Verification items for the finished model (mm, model axes). Face numbers are marked on the shaded views. Give positions to 0.01 mm unless a question says otherwise; leave off trailing zeros. Write each loop counter-clockwise with the first axis right and the second up, starting at its lowest first coordinate (ties: lowest second). Pieces come first, ordered by that corner, then holes. Notation, with made-up numbers: (-38.5, -26.5) -> (-23.5, -26.5) arc R21 ccw to (-23.5, -10.5) -> close; hole circle Ø5 at (-25.5, 21.25). An arc over 180 degrees is marked (long way). Write item = value, one per line.
from build123d import *

# Parameters (mm, degrees)
BOSS_EXTRUDE1_DEPTH = 6.1
BOSS_EXTRUDE4_START = -5
BOSS_EXTRUDE4_DEPTH = 5
BOSS_EXTRUDE5_START = 5
SKETCH6_R           = 2.75
BOSS_EXTRUDE5_DEPTH = 5
SKETCH7_R           = 2.75
CUT_EXTRUDE1_DEPTH  = 176.534516689


with BuildPart() as part:
    # Sketch4 → Boss-Extrude1 (new body)
    with BuildSketch(Plane.XY):
        with BuildLine():
            Line((2.791805242, 138.827155544), (104.55323324, 91.375022364))
            Line((104.55323324, 91.375022364), (105.415210237, 92.128353131))
            ThreePointArc((105.415210237, 92.128353131), (9.395226761, 139.684393237), (-92.128353131, 105.415210237))
            Line((-92.128353131, 105.415210237), (-91.375022364, 104.55323324))
            Line((-91.375022364, 104.55323324), (2.791805242, 138.827155544))
        make_face()
    extrude(amount=BOSS_EXTRUDE1_DEPTH)

    # Sketch5 → Boss-Extrude4 (add)
    with BuildSketch(Plane.XY.offset(BOSS_EXTRUDE4_START)):
        with BuildLine():
            Line((30.722164617, 125.803015072), (76.622873865, 104.399162835))
            ThreePointArc((76.622873865, 104.399162835), (87.59255508, 95.382358403), (97.50906947, 85.218726646))
            Line((97.50906947, 85.218726646), (105.415210237, 92.128353131))
            ThreePointArc((105.415210237, 92.128353131), (9.395226761, 139.684393237), (-92.128353131, 105.415210237))
            Line((-92.128353131, 105.415210237), (-85.218726646, 97.50906947))
            ThreePointArc((-85.218726646, 97.50906947), (-30.701883618, 125.807966132), (30.722164617, 125.803015072))
        make_face()
    extrude(amount=BOSS_EXTRUDE4_DEPTH)

    # Sketch6 → Boss-Extrude5 (add)
    with BuildSketch(Plane(origin=(0, 0, -5), x_dir=(-1, 0, 0), z_dir=(0, 0, -1)).offset(BOSS_EXTRUDE5_START)):
        with BuildLine():
            Line((-10, 129.5), (10, 129.5))
            Line((10, 129.5), (10, 109.268365161))
            ThreePointArc((10, 109.268365161), (43.208620922, 100.85926186), (72.205596766, 82.619171024))
            Line((72.205596766, 82.619171024), (92.128353131, 105.415210237))
            ThreePointArc((92.128353131, 105.415210237), (-9.395226761, 139.684393237), (-105.415210237, 92.128353131))
            Line((-105.415210237, 92.128353131), (-82.619171024, 72.205596766))
            ThreePointArc((-82.619171024, 72.205596766), (-49.879754516, 97.732214313), (-10, 109.268365161))
            Line((-10, 109.268365161), (-10, 129.5))
        make_face()
        with Locations((54.966796439, 107.162966034)):
            Circle(SKETCH6_R, mode=Mode.SUBTRACT)
    extrude(amount=-BOSS_EXTRUDE5_DEPTH)

    # Sketch7 → Cut-Extrude1 (cut, through all)
    with BuildSketch(Plane.XY):
        with Locations((76.813119358, 91.542310953)):
            Circle(SKETCH7_R)
    extrude(amount=-CUT_EXTRUDE1_DEPTH, mode=Mode.SUBTRACT)


solid = part.part
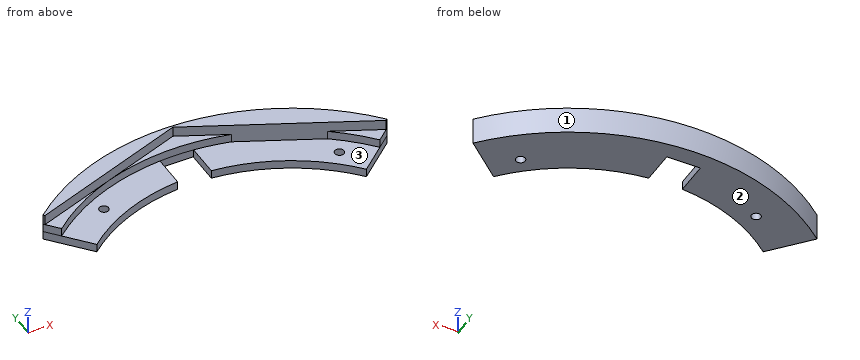
Item 1: Sectioned sample at B-B on z = 2. Record the cut outline in (x, y).
Response values:
outline = (-92.13, 105.42) -> (-91.38, 104.55) -> (2.79, 138.83) -> (104.55, 91.38) -> (105.42, 92.13) arc R140 ccw to start
Item 2: Go/stop test with flat-tipped pins: P1, Ø1.5, axis at y = 123.5, z = -7.5, coming from the -X side; P2, Ø4, axis at x = 0.5, z = -7, coming from the -Y side; P3, Ø5, axis at x = 6.5, y = 128, coming from the +Z side. Record where each tip stops, or that it passes through.
Response values:
P1 = -67.32
P2 = 129.5
P3 = 0
Item 3: Mould release check, pull along X, two halves, no side actions. Record for the marked faces 1, 2 and 3: +X half, -X half, draft (parallel to the pull), parting line (faces both ways), or undercut.
Response values:
face_1 = parting line
face_2 = draft
face_3 = undercut
Item 4: Sectioned sample at D-D on y = 134. Record the cut outline in (x, z), then the cut area to 3 significant figures.
Response values:
outline = (-40.55, -10) -> (40.55, -10) -> (40.55, 6.1) -> (13.14, 6.1) -> (13.14, 0) -> (-10.47, 0) -> (-10.47, 6.1) -> (-40.55, 6.1) -> close
area = 1,160 mm^2
Item 5: Sectioned sample at C-C on x = 22. Record the cut outline in (y, z), then the cut area to 3 significant figures.
Response values:
outline = (107.5, -10) -> (138.26, -10) -> (138.26, 6.1) -> (129.87, 6.1) -> (129.87, 0) -> (127.62, 0) -> (127.62, -5) -> (107.5, -5) -> close
area = 258 mm^2
Item 6: Material ranges on line 1 (X direction, y = 103, z = -0.25); line 2 (Z direction, x = -23, y = 121.5); line 3 (X direction, y = 115, z = -0.5), recorded low to high.
Response values:
line_1 = -90.02 to -78.49, 78.49 to 94.82
line_2 = -10 to -5
line_3 = -79.84 to -59.54, 53.89 to 79.84
Item 7: Sectioned sample at A-A on y = 114. Record the cut outline in (x, z) (3 decimals), then the cut area to 3 significant figures.
Response values:
outline = (-81.265, -10) -> (-10, -10) -> (-10, -5) -> (-61.435, -5) -> (-61.435, 0) -> (-65.42, 0) -> (-65.42, 6.1) -> (-81.265, 6.1) -> close; (10, -10) -> (81.265, -10) -> (81.265, 6.1) -> (56.034, 6.1) -> (56.034, -5) -> (10, -5) -> close
area = 1,190 mm^2
